The model under review builds one solid part; all positions refer to its coordinate system, in mm. A direction names the side the tool comes from. Give positions to 0.01 mm unless a question says otherwise; leave off trailing zeros. Loops run counter-clockwise (first coordinate to the right, second up) from the corner with the lowest first, then second, coordinate; pieces in that order, holes last. Notation, with made-up numbers: (75, 44.25) -> (130, 44.25) arc R22 cw to (130, 83.25) -> close; hole circle Ø4 at (64.5, 66). An arc over 180 degrees is marked (long way). Write each question's results on one line, items separated by ' | '. Start each with the question number.
Q1. Wall thickness on L1, parallel to X at y = 2.65, z = 0; L2, parallel to Y at x = 10, z = 1.5; L3, parallel to X at y = 3.25, z = 2.75: over which ranges is each line inside the solid? List them lowest first. Write a range as [from, to].
Q2. We need section A-A (x = -8). Write out the cut boundary in (y, z), plus the area to 3 significant figures.
Q3. Machinability: for faces 4 (the face through (6, 0.5, 1)), 5 (the face through (-10.83, 2.55, 0.15)), which of the approach directions +Z, -Z, +X, -X, +Y, -Y give a long, thin tool a straight path to every point of the face, cutting with its end or side? Answer none if there is none.
Q4. Insertion check: pin 1 Ø2.5 at (x, z) = (12, 0) entering from +Y; pin 2 Ø6 at (x, y) = (-9, 2.5) entering from -Z; pin 3 Ø3 at (x, z) = (-12, 0) entering from -Y; pin 4 Ø2 at (x, z) = (8, 0) entering from -Y. Each pin has a flat end and moves straight along its axis. Give the tip position at first contact, or say it passes through.
Q5. We need section C-C (y = 11). Write out the cut boundary in (x, z), plus the area to 3 significant figures.
Q6. Mouldability with a two-part tool opening along Z and no side actions: class faces 1 (the face through (14.85, 0.25, 0.05)), 2 (the face through (2, 0, 0)), 3 (the face through (0, 3.05, 0)) as released by +Z, released by -Z, zero draft, split by the parting line, or undercut.
Q7. We need section B-B (y = 15.5). Write out the cut boundary in (x, z), plus the area to 3 significant figures.
from build123d import *

# Parameters (mm, degrees)
SKETCH2_R           = 1.18
BOSS_EXTRUDE1_DEPTH = 0.5
SKETCH3_R           = 1.18
BOSS_EXTRUDE2_DEPTH = 0.5
CUT_EXTRUDE1_DEPTH  = 10
CIRPATTERN1_COUNT   = 2
CIRPATTERN1_ANGLE   = 180


with BuildPart() as part:
    # Sketch1 → Revolve1 (revolve)
    with BuildSketch(Plane.XY, mode=Mode.PRIVATE) as revolve1_sk:
        with BuildLine():
            Line((5.5, 20.3), (5.5, 3.8))
            ThreePointArc((5.5, 3.8), (5.207106781, 3.092893219), (4.5, 2.8))
            Line((4.5, 2.8), (5.5, 2.8))
            Line((5.5, 2.8), (5.5, 2.3))
            Line((5.5, 2.3), (5, 2.3))
            Line((5, 2.3), (5, 0.5))
            Line((5, 0.5), (5.5, 0.5))
            Line((5.5, 0.5), (5.5, 0))
            Line((5.5, 0), (0, 0))
            Line((0, 0), (0, 3.05))
            Line((0, 3.05), (4.5, 3.05))
            ThreePointArc((4.5, 3.05), (5.030330086, 3.269669914), (5.25, 3.8))
            Line((5.25, 3.8), (5.25, 20.3))
            Line((5.25, 20.3), (5.5, 20.3))
        make_face()
    revolve(revolve1_sk.sketch.rotate(Axis((0, -2.4, 0), (0, 1, 0)), 90), axis=Axis((0, -2.4, 0), (0, 1, 0)))

    # Sketch2 → Boss-Extrude1 (add)
    with BuildSketch(Plane.XZ):
        with BuildLine():
            Line((5.018714975, 2.25), (12.6, 2.25))
            ThreePointArc((12.6, 2.25), (14.85, 0), (12.6, -2.25))
            Line((12.6, -2.25), (5.018714975, -2.25))
            ThreePointArc((5.018714975, -2.25), (5.5, 0), (5.018714975, 2.25))
        make_face()
        with Locations(Location((12, 0, 0), (0, 0, 270))):
            Circle(SKETCH2_R, mode=Mode.SUBTRACT)
        with Locations(Location((8, 0, 0), (0, 0, 270))):
            Circle(SKETCH2_R, mode=Mode.SUBTRACT)
    extrude(amount=-BOSS_EXTRUDE1_DEPTH)

    # Sketch3 → Boss-Extrude2 (add)
    with BuildSketch(Plane.XZ.offset(-2.3)):
        with BuildLine():
            Line((-5.018714975, 2.25), (-12.6, 2.25))
            ThreePointArc((-12.6, 2.25), (-14.85, 0), (-12.6, -2.25))
            Line((-12.6, -2.25), (-5.018714975, -2.25))
            ThreePointArc((-5.018714975, -2.25), (-5.37833303, -1.150449399), (-5.5, 0))
            ThreePointArc((-5.5, 0), (-5.37833303, 1.150449399), (-5.018714975, 2.25))
        make_face()
        with Locations(Location((-12, 0, 0), (0, 0, 270))):
            Circle(SKETCH3_R, mode=Mode.SUBTRACT)
        with Locations(Location((-8, 0, 0), (0, 0, 270))):
            Circle(SKETCH3_R, mode=Mode.SUBTRACT)
    extrude(amount=-BOSS_EXTRUDE2_DEPTH)

    # Sketch4 → Cut-Extrude1 (cut)
    with BuildSketch(Plane(origin=(0, 0, 0), x_dir=(0, 0, -1), z_dir=(1, 0, 0))):
        with BuildLine():
            Line((2.298813226, 20.3), (2.298813226, 15.95))
            ThreePointArc((2.298813226, 15.95), (2.005920007, 15.242893219), (1.298813226, 14.95))
            Line((1.298813226, 14.95), (-1.283627995, 14.95))
            ThreePointArc((-1.283627995, 14.95), (-2.351186774, 16.017558779), (-1.283627995, 17.085117557))
            ThreePointArc((-1.283627995, 17.085117557), (-1.03323034, 17.046337207), (-0.806294362, 16.933629784))
            ThreePointArc((-0.806294362, 16.933629784), (-0.079626551, 16.883947504), (0.298813226, 17.506280029))
            Line((0.298813226, 17.506280029), (0.298813226, 20.3))
            Line((0.298813226, 20.3), (2.298813226, 20.3))
        make_face()
    cut_extrude1 = extrude(amount=CUT_EXTRUDE1_DEPTH, mode=Mode.SUBTRACT)

    # CirPattern1: Cut-Extrude1 ×2 about axis
    cirpattern1_axis = Axis((0, 20.3, 0), (0, -1, 0))
    for i in range(1, CIRPATTERN1_COUNT):
        add(cut_extrude1.rotate(cirpattern1_axis, i * CIRPATTERN1_ANGLE / (CIRPATTERN1_COUNT - 1)), mode=Mode.SUBTRACT)


solid = part.part
Output:
1) L1: [-14.85, -13.18], [-10.82, -9.18], [-6.82, 5.5] | L2: [0, 0.5] | L3: [-4.57, -4.19], [4.19, 4.57]
2) outline: (2.3, -2.25) -> (2.8, -2.25) -> (2.8, -1.18) -> (2.3, -1.18) -> close; (2.3, 1.18) -> (2.8, 1.18) -> (2.8, 2.25) -> (2.3, 2.25) -> close | area: 1.07 mm2
3) face 4: none | face 5: +Y, -Y
4) pin 1: y = 0.5 | pin 2: z = -2.25 | pin 3: y = 2.3 | pin 4: through
5) outline: circle Ø11 at (0, 0); hole circle Ø10.5 at (0, 0) | area: 8.44 mm2
6) face 1: split by the parting line | face 2: zero draft | face 3: undercut
7) outline: (-5.04, 2.19) -> (-4.77, 2.19) arc R5.25 cw to (4.76, 2.22) -> (5.03, 2.22) arc R5.5 ccw to start; (-5.03, -2.22) arc R5.5 ccw to (5.04, -2.19) -> (4.77, -2.19) arc R5.25 cw to (-4.76, -2.22) -> close | area: 6.17 mm2
